Here's how the part is built. I have some questions about the finished solid (model axes, mm). Coordinates: 2 decimals unless noted, no trailing zeros. Loops run counter-clockwise (first coordinate to the right, second up) from the corner with the lowest first, then second, coordinate; pieces in that order, holes last. Notation, with made-up numbers: (13, -31) -> (24, -31) arc R27 ccw to (24, 1) -> close; hole circle Ø6 at (72.25, 11). An arc over 180 degrees is marked (long way). Answer as a JSON object with one key per item and string values. Group by question number.
1) I'm going to push flat-ended pins straight in: pin 1 (12 mm diameter, centred on y = 5.5, z = 11.5, fed in from -X); pin 2 (4 mm diameter, centred on y = 0, z = 0, fed in from +X); pin 3 (6 mm diameter, centred on y = -5, z = -25, fed in from +X). Where does each tip first touch, or does it pass through?
2) I need wall thicknesses on probe 1 along Z at (x, y) = (1.5, 4); probe 2 along Z at (x, y) = (0.25, 0); probe 3 along Y at (x, z) = (1.2, -14). Which ranges of each line are inside material? Lowest first, please. Write a range as [from, to].
3) I want a section at A-A (y = 0). Write out the boundary of the cut face in (x, z).
4) I want a section at D-D (z = -8). Write out the boundary of the cut face in (x, y).
5) I want a section at C-C (y = 4). Write out the boundary of the cut face in (x, z).
6) I want a section at B-B (z = 0). Write out the boundary of the cut face in (x, y), then the cut area to 3 significant figures.
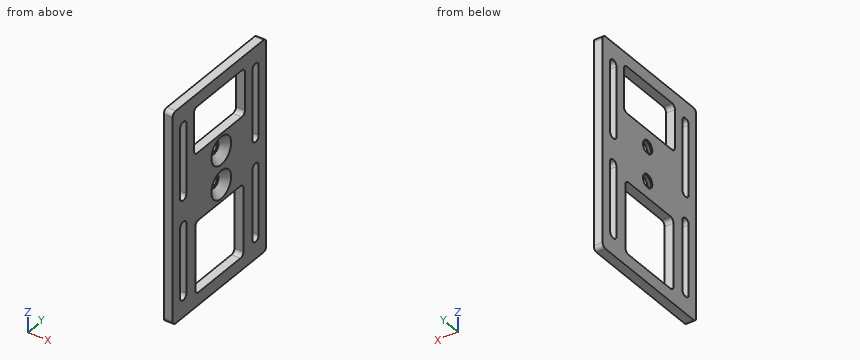
```python
from build123d import *

# Parameters (mm, degrees)
SKETCH_1_W               = 50
SKETCH_1_H               = 31.2
SKETCH_1_R               = 1.55
SKETCH_1_W_2             = 18.5
SKETCH_1_H_2             = 2.1
SKETCH_1_W_3             = 17
SKETCH_1_H_3             = 16
SKETCH_1_W_4             = 11
SKETCH_1_H_4             = 17
EXTRUDE_1_DEPTH          = 2.1
HOLE_WIZARD_1_AT_2_COUNT = 2
HOLE_WIZARD_1_AT_2_PITCH = 8
FILLET_1_R               = 1


with BuildPart() as part:
    # 草图1 → 凸台-拉伸1 (new body)
    with BuildSketch(Plane(origin=(0, 0, 0), x_dir=(0, 0, -1), z_dir=(1, 0, 0))):
        with Locations((7, -0.6)):
            Rectangle(SKETCH_1_W, SKETCH_1_H)
        Circle(SKETCH_1_R, mode=Mode.SUBTRACT)
        with Locations((8, 0)):
            Circle(SKETCH_1_R, mode=Mode.SUBTRACT)
        with Locations((-4.75, 11.45)):
            Rectangle(SKETCH_1_W_2, SKETCH_1_H_2, mode=Mode.SUBTRACT)
        with Locations((18.75, 11.45)):
            Rectangle(SKETCH_1_W_2, SKETCH_1_H_2, mode=Mode.SUBTRACT)
        with Locations((18.75, -12.65)):
            Rectangle(SKETCH_1_W_2, SKETCH_1_H_2, mode=Mode.SUBTRACT)
        with Locations((-4.75, -12.65)):
            Rectangle(SKETCH_1_W_2, SKETCH_1_H_2, mode=Mode.SUBTRACT)
        with Locations((20.5, -0.6)):
            Rectangle(SKETCH_1_W_3, SKETCH_1_H_3, mode=Mode.SUBTRACT)
        with Locations((-9.5, -0.6)):
            Rectangle(SKETCH_1_W_4, SKETCH_1_H_4, mode=Mode.SUBTRACT)
    extrude(amount=EXTRUDE_1_DEPTH)

    # 草图2 → 打孔尺寸(%根据十字)槽沉头木螺钉的类型1 (revolve, cut)
    with BuildSketch(Plane(origin=(2.1, 0, 0), x_dir=(0, 0, -1), z_dir=(0, 1, 0))):
        Polygon((0, 0), (0, 2.1), (1.55, 2.1), (1.55, 1.75), (3.3, 0), align=None)
    hole_wizard_1 = revolve(axis=Axis((8.45, 0, 0), (-1, 0, 0)), mode=Mode.SUBTRACT)

    # 打孔尺寸(%根据十字)槽沉头木螺钉的类型1 at 2: 打孔尺寸(%根据十字)槽沉头木螺钉的类型1 ×2
    with Locations(*[(0, 0, -i * HOLE_WIZARD_1_AT_2_PITCH) for i in range(1, HOLE_WIZARD_1_AT_2_COUNT)]):
        add(hole_wizard_1, mode=Mode.SUBTRACT)

    # 圆角1
    fillet_1_edges = [part.edges().sort_by_distance(p)[0] for p in [
        (1.05, 12.5, 14),
        (1.05, 10.4, 14),
        (1.05, 10.4, -4.5),
        (1.05, 12.5, -4.5),
        (1.05, 12.5, -9.5),
        (1.05, 10.4, -9.5),
        (1.05, 10.4, -28),
        (1.05, 12.5, -28),
        (1.05, -11.6, -28),
        (1.05, -11.6, -9.5),
        (1.05, -13.7, -9.5),
        (1.05, -13.7, -28),
        (1.05, -13.7, -4.5),
        (1.05, -11.6, -4.5),
        (1.05, -11.6, 14),
        (1.05, -13.7, 14),
        (1.05, 15, 18),
        (1.05, 7.4, -12),
        (1.05, 15, -32),
        (1.05, -8.6, -12),
        (1.05, -8.6, -29),
        (1.05, 7.4, -29),
        (1.05, -16.2, -32),
        (1.05, -16.2, 18),
        (1.05, 7.9, 15),
        (1.05, -9.1, 15),
        (1.05, -9.1, 4),
        (1.05, 7.9, 4),
    ]]
    fillet(fillet_1_edges, radius=FILLET_1_R)


solid = part.part
```
Determined:
{
 "1": {"pin 1": "x = 0", "pin 2": "x = 0.8", "pin 3": "through"},
 "2": {"probe 1": "[-32, -29], [-12, 4], [15, 18]", "probe 2": "[-32, -29], [-12, -9.55], [-6.45, -1.55], [1.55, 4], [15, 18]", "probe 3": "[-16.2, -13.7], [-11.6, -8.6], [7.4, 10.4], [12.5, 15]"},
 "3": {"outline": "(0, -32) -> (2.1, -32) -> (2.1, -29) -> (0, -29) -> close; (0, -12) -> (2.1, -12) -> (2.1, -11.3) -> (0.35, -9.55) -> (0, -9.55) -> close; (0, -6.45) -> (0.35, -6.45) -> (2.1, -4.7) -> (2.1, -3.3) -> (0.35, -1.55) -> (0, -1.55) -> close; (0, 1.55) -> (0.35, 1.55) -> (2.1, 3.3) -> (2.1, 4) -> (0, 4) -> close; (0, 15) -> (2.1, 15) -> (2.1, 18) -> (0, 18) -> close"},
 "4": {"outline": "(0, -16.2) -> (2.1, -16.2) -> (2.1, -3.3) -> (0.35, -1.55) -> (0, -1.55) -> close; (0, 1.55) -> (0.35, 1.55) -> (2.1, 3.3) -> (2.1, 15) -> (0, 15) -> close"},
 "5": {"outline": "(0, -32) -> (2.1, -32) -> (2.1, -29) -> (0, -29) -> close; (0, -12) -> (2.1, -12) -> (2.1, 4) -> (0, 4) -> close; (0, 15) -> (2.1, 15) -> (2.1, 18) -> (0, 18) -> close"},
 "6": {"outline": "(0, -16.2) -> (2.1, -16.2) -> (2.1, -13.7) -> (0, -13.7) -> close; (0, -11.6) -> (2.1, -11.6) -> (2.1, -3.3) -> (0.35, -1.55) -> (0, -1.55) -> close; (0, 1.55) -> (0.35, 1.55) -> (2.1, 3.3) -> (2.1, 10.4) -> (0, 10.4) -> close; (0, 12.5) -> (2.1, 12.5) -> (2.1, 15) -> (0, 15) -> close", "area": "47.1 mm^2"}
}
